```python
from build123d import *

# Parameters (mm, degrees)
F0_R     = 57.15
F3_T     = -6
F4_DEPTH = 25
F5_R     = 57.15
F5_R_2   = 51.15
F6_DEPTH = 25


with BuildPart() as f2:
    # F2: sweep along a path in F1
    with BuildLine(Plane.XZ) as f2_path:
        ThreePointArc((152, 152), (44.5197692596, 107.4802307404), (0, 0))
    # F0 (on Top) → F2 (sweep)
    with BuildSketch(Plane.XY):
        Circle(F0_R)
    sweep(path=f2_path.line)

    # F3
    f3_openings = [f2.faces().sort_by_distance(p)[0] for p in [
        (152, 0, 152),
        (0, 0, 0),
    ]]
    offset(amount=F3_T, openings=f3_openings, kind=Kind.INTERSECTION)

    # F0 (on Top) → F4 (join)
    with BuildSketch(Plane.XY):
        Circle(F0_R)
    extrude(amount=-F4_DEPTH)

    # F5 (on face) → F6 (join)
    with BuildSketch(Plane.YZ.offset(152)):
        with Locations((0, 152)):
            Circle(F5_R)
        with Locations((0, 152)):
            Circle(F5_R_2, mode=Mode.SUBTRACT)
    extrude(amount=F6_DEPTH)


solid = f2.part
```
Verification items for the finished model (mm, model axes). Coordinates: 2 decimals unless noted, no trailing zeros. Loops run counter-clockwise (first coordinate to the right, second up) from the corner with the lowest first, then second, coordinate; pieces in that order, holes last. Notation, with made-up numbers: (0, 20) - (5, 20) arc R25 cw to (5, 51) - close; hole circle Ø1 at (74, 20). An arc over 180 degrees is marked (long way). Answer as a JSON object with one key per item and string values.
(1) Scan lines: line 1 along Z through (x, y) = (167, 0); line 2 along Y through (x, z) = (1.5, 8.5); line 3 along X through (y, z) = (9, 32). Record each from-to range of solid material in increasing order.
Response:
{"line 1": "z = 94.85 to 100.85, 203.15 to 209.15", "line 2": "y = -57.14 to -51.13, 51.13 to 57.14", "line 3": "x = -53.97 to -47.81, 55.52 to 61.95"}
(2) Mould release check, pull along X, two halves, no side actions. Record for faces 1 (the flat face through (-1, 1, 0)), 2 (the flat face through (177, -43, 123)), 3 (the flat face through (-1, 1, -25)), 4 (the cylindrical face through (-57.095, 2.513, -12.325)): pulls with the +X half, pulls with the -X half, needs draft (parallel to the pull), parting line crosses it, or undercut.
Response:
{"face 1": "undercut", "face 2": "pulls with the +X half", "face 3": "needs draft", "face 4": "parting line crosses it"}
(3) Go/stop test with flat-tipped pins: pin 1 Ø3 at (x, z) = (106.5, 161) entering from +Y; pin 2 Ø5 at (y, z) = (42.5, 6) entering from -X; pin 3 Ø1 at (x, z) = (6, 130.5) entering from +Y. Record where each tip stops, or that it passes through.
Response:
{"pin 1": "stops at y = 55.46", "pin 2": "stops at x = -40.73", "pin 3": "stops at y = 37.27"}
(4) Cross-section at A-A, the plane y = 0. Record the boundary of the cut face in (x, z), then the cut area to 3 significant figures.
Response:
{"outline": "(-57.15, -25) - (57.15, -25) - (57.15, 0) arc R94.85 cw to (152, 94.85) - (177, 94.85) - (177, 100.85) - (152, 100.85) arc R100.85 ccw to (51.15, 0) - (-51.15, 0) arc R203.15 cw to (152, 203.15) - (177, 203.15) - (177, 209.15) - (152, 209.15) arc R209.15 ccw to (-57.15, 0) - close", "area": "6,020 mm²"}
(5) Cross-section at B-B, the plane y = -31.5. Record the boundary of the cut face in (x, z), then the cut area to 3 significant figures.
Response:
{"outline": "(-47.69, -25) - (47.69, -25) - (47.69, 0) arc R104.31 cw to (152, 104.31) - (177, 104.31) - (177, 111.7) - (152, 111.7) arc R111.7 ccw to (40.3, 0) - (-40.3, 0) arc R192.3 cw to (152, 192.3) - (177, 192.3) - (177, 199.69) - (152, 199.69) arc R199.69 ccw to (-47.69, 0) - close", "area": "6,280 mm²"}
